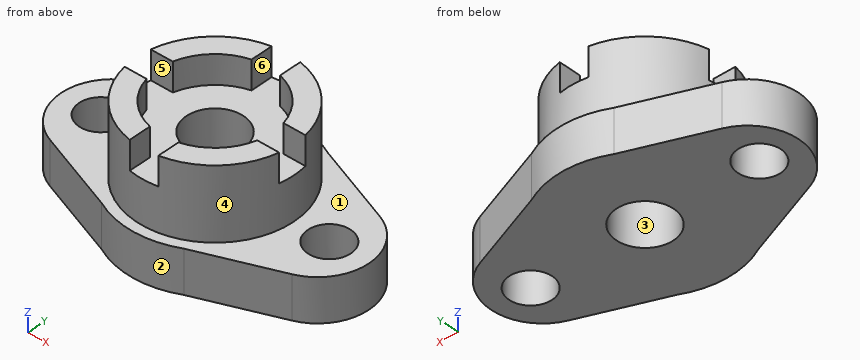
```python
from build123d import *

# Parameters (mm, degrees)
F1_DEPTH = 19.05
F2_DEPTH = 38.1
F3_R     = 34.925
F3_R_2   = 12.7
F4_DEPTH = 12.7
F6_DEPTH = 12.7
F0_R     = 9.525
F7_DEPTH = 19.05
F8_DEPTH = 103.378
F9_DEPTH = 38.1


# Not quite as in the source:
# - a feature names something its author has since deleted; it is built from what else it names


with BuildPart() as f1:
    # F0 (on Top) → F1 (new body)
    with BuildSketch(Plane.XY):
        with BuildLine():
            ThreePointArc((-34.925, 0), (0, -34.925), (34.925, 0))
            Line((34.925, 0), (25.4, 0))
            ThreePointArc((25.4, 0), (0, -25.4), (-25.4, 0))
            Line((-25.4, 0), (-34.925, 0))
        make_face()
        with BuildLine():
            Line((25.4, 0), (34.925, 0))
            ThreePointArc((34.925, 0), (0, 34.925), (-34.925, 0))
            Line((-34.925, 0), (-25.4, 0))
            ThreePointArc((-25.4, 0), (0, 25.4), (25.4, 0))
        make_face()
    extrude(amount=F1_DEPTH)

    # F0 (on Top) → F2 (join)
    with BuildSketch(Plane.XY):
        with BuildLine():
            ThreePointArc((-34.925, 0), (0, -34.925), (34.925, 0))
            Line((34.925, 0), (25.4, 0))
            ThreePointArc((25.4, 0), (0, -25.4), (-25.4, 0))
            Line((-25.4, 0), (-34.925, 0))
        make_face()
        with BuildLine():
            Line((25.4, 0), (34.925, 0))
            ThreePointArc((34.925, 0), (0, 34.925), (-34.925, 0))
            Line((-34.925, 0), (-25.4, 0))
            ThreePointArc((-25.4, 0), (0, 25.4), (25.4, 0))
        make_face()
        with BuildLine():
            ThreePointArc((-25.4, 0), (0, -25.4), (25.4, 0))
            Line((25.4, 0), (12.7, 0))
            ThreePointArc((12.7, 0), (0, -12.7), (-12.7, 0))
            Line((-12.7, 0), (-25.4, 0))
        make_face()
        with BuildLine():
            Line((12.7, 0), (25.4, 0))
            ThreePointArc((25.4, 0), (0, 25.4), (-25.4, 0))
            Line((-25.4, 0), (-12.7, 0))
            ThreePointArc((-12.7, 0), (0, 12.7), (12.7, 0))
        make_face()
    extrude(amount=F2_DEPTH)

    # F3 (on face) → F4 (join)
    with BuildSketch(Plane.XY.offset(38.1)):
        Circle(F3_R)
        Circle(F3_R_2, mode=Mode.SUBTRACT)
    extrude(amount=F4_DEPTH)

    # F5 (on face) → F6 (cut)
    with BuildSketch(Plane.XY.offset(50.8)):
        with BuildLine():
            ThreePointArc((-24.5934442484, -6.35), (-25.4, 0), (-24.5934442484, 6.35))
            Line((-24.5934442484, 6.35), (-34.3428758988, 6.35))
            ThreePointArc((-34.3428758988, 6.35), (-34.925, 0), (-34.3428758988, -6.35))
            Line((-34.3428758988, -6.35), (-24.5934442484, -6.35))
        make_face()
        with BuildLine():
            Line((6.35, -34.3428758988), (6.35, -24.5934442484))
            ThreePointArc((6.35, -24.5934442484), (0, -25.4), (-6.35, -24.5934442484))
            Line((-6.35, -24.5934442484), (-6.35, -34.3428758988))
            ThreePointArc((-6.35, -34.3428758988), (0, -34.925), (6.35, -34.3428758988))
        make_face()
        with BuildLine():
            Line((34.3428758988, 6.35), (24.5934442484, 6.35))
            ThreePointArc((24.5934442484, 6.35), (25.1975542852, 3.2005090291), (25.4, 0))
            ThreePointArc((25.4, 0), (25.1975542852, -3.2005090291), (24.5934442484, -6.35))
            Line((24.5934442484, -6.35), (34.3428758988, -6.35))
            ThreePointArc((34.3428758988, -6.35), (34.7791644937, -3.1883133656), (34.925, 0))
            ThreePointArc((34.925, 0), (34.7791644937, 3.1883133656), (34.3428758988, 6.35))
        make_face()
        with BuildLine():
            ThreePointArc((-6.35, 24.5934442484), (0, 25.4), (6.35, 24.5934442484))
            Line((6.35, 24.5934442484), (6.35, 34.3428758988))
            ThreePointArc((6.35, 34.3428758988), (0, 34.925), (-6.35, 34.3428758988))
            Line((-6.35, 34.3428758988), (-6.35, 24.5934442484))
        make_face()
    extrude(amount=-F6_DEPTH, mode=Mode.SUBTRACT)

    # F0 (on Top) → F7 (join)
    with BuildSketch(Plane.XY):
        with BuildLine():
            Line((53.7687589873, 21.2442149995), (18.2328532376, 34.9850083733))
            ThreePointArc((18.2328532376, 34.9850083733), (0, 39.4510804423), (-18.2328532376, 34.9850083733))
            Line((-18.2328532376, 34.9850083733), (-53.7687589873, 21.2442149995))
            ThreePointArc((-53.7687589873, 21.2442149995), (-68.3312757395, 0), (-53.7687589873, -21.2442149995))
            Line((-53.7687589873, -21.2442149995), (-18.2328532376, -34.9850083733))
            ThreePointArc((-18.2328532376, -34.9850083733), (0, -39.4510804423), (18.2328532376, -34.9850083733))
            Line((18.2328532376, -34.9850083733), (53.7687589873, -21.2442149995))
            ThreePointArc((53.7687589873, -21.2442149995), (68.3312757395, 0), (53.7687589873, 21.2442149995))
        make_face()
        with Locations((-50.8, 0)):
            Circle(F0_R, mode=Mode.SUBTRACT)
        with BuildLine():
            ThreePointArc((-34.925, 0), (0, 34.925), (34.925, 0))
            ThreePointArc((34.925, 0), (0, -34.925), (-34.925, 0))
        make_face(mode=Mode.SUBTRACT)
        with BuildLine():
            ThreePointArc((60.325, 0), (50.8, -9.525), (41.275, 0))
            ThreePointArc((41.275, 0), (50.8, 9.525), (60.325, 0))
        make_face(mode=Mode.SUBTRACT)
    extrude(amount=F7_DEPTH)

    # F5 (on face) → F8 (cut)
    with BuildSketch(Plane.XY.offset(50.8)):
        with BuildLine():
            Line((6.35, 6.35), (6.35, 0))
            Line((6.35, 0), (6.35, -6.35))
            Line((6.35, -6.35), (24.5934442484, -6.35))
            ThreePointArc((24.5934442484, -6.35), (25.1975542852, -3.2005090291), (25.4, 0))
            ThreePointArc((25.4, 0), (25.1975542852, 3.2005090291), (24.5934442484, 6.35))
            Line((24.5934442484, 6.35), (6.35, 6.35))
        make_face()
        with BuildLine():
            Line((-6.35, -6.35), (-6.35, 0))
            Line((-6.35, 0), (-6.35, 6.35))
            Line((-6.35, 6.35), (-24.5934442484, 6.35))
            ThreePointArc((-24.5934442484, 6.35), (-25.4, 0), (-24.5934442484, -6.35))
            Line((-24.5934442484, -6.35), (-6.35, -6.35))
        make_face()
        with BuildLine():
            Line((-6.35, 6.35), (0, 6.35))
            Line((0, 6.35), (6.35, 6.35))
            Line((6.35, 6.35), (6.35, 24.5934442484))
            ThreePointArc((6.35, 24.5934442484), (0, 25.4), (-6.35, 24.5934442484))
            Line((-6.35, 24.5934442484), (-6.35, 6.35))
        make_face()
        with BuildLine():
            Line((6.35, -6.35), (0, -6.35))
            Line((0, -6.35), (-6.35, -6.35))
            Line((-6.35, -6.35), (-6.35, -24.5934442484))
            ThreePointArc((-6.35, -24.5934442484), (0, -25.4), (6.35, -24.5934442484))
            Line((6.35, -24.5934442484), (6.35, -6.35))
        make_face()
        with BuildLine():
            Line((6.35, 24.5934442484), (6.35, 6.35))
            Line((6.35, 6.35), (24.5934442484, 6.35))
            ThreePointArc((24.5934442484, 6.35), (17.9605122421, 17.9605122421), (6.35, 24.5934442484))
        make_face()
        with BuildLine():
            Line((24.5934442484, -6.35), (6.35, -6.35))
            Line((6.35, -6.35), (6.35, -24.5934442484))
            ThreePointArc((6.35, -24.5934442484), (17.9605122421, -17.9605122421), (24.5934442484, -6.35))
        make_face()
        with BuildLine():
            Line((-24.5934442484, 6.35), (-6.35, 6.35))
            Line((-6.35, 6.35), (-6.35, 24.5934442484))
            ThreePointArc((-6.35, 24.5934442484), (-17.9605122421, 17.9605122421), (-24.5934442484, 6.35))
        make_face()
        with BuildLine():
            Line((-6.35, -24.5934442484), (-6.35, -6.35))
            Line((-6.35, -6.35), (-24.5934442484, -6.35))
            ThreePointArc((-24.5934442484, -6.35), (-17.9605122421, -17.9605122421), (-6.35, -24.5934442484))
        make_face()
    extrude(amount=-F8_DEPTH, mode=Mode.SUBTRACT)

    # F0 (on Top) → F9 (join)
    with BuildSketch(Plane.XY):
        with BuildLine():
            ThreePointArc((-25.4, 0), (0, -25.4), (25.4, 0))
            Line((25.4, 0), (12.7, 0))
            ThreePointArc((12.7, 0), (0, -12.7), (-12.7, 0))
            Line((-12.7, 0), (-25.4, 0))
        make_face()
        with BuildLine():
            Line((12.7, 0), (25.4, 0))
            ThreePointArc((25.4, 0), (0, 25.4), (-25.4, 0))
            Line((-25.4, 0), (-12.7, 0))
            ThreePointArc((-12.7, 0), (0, 12.7), (12.7, 0))
        make_face()
    extrude(amount=F9_DEPTH)


solid = f1.part
```
Design review of the part built by this model. Coordinates are the model's own, in mm. Face numbers are marked on the shaded views. A direction names the side the tool comes from. Coordinates: 2 decimals unless noted, no trailing zeros. Write each loop counter-clockwise with the first axis right and the second up, starting at its lowest first coordinate (ties: lowest second). Pieces come first, ordered by that corner, then holes. Notation, with made-up numbers: M 63.5,79.5 L 68.5,79.5 A25 ccw 68.5,114.5 Z; hole C -13,31 d10. An arc over 180 degrees is marked long. Answer as a JSON object with one key per item and string values.
Item 1: Add section B-B, the plane x = 0. Give the boundary of the cut face in (y, z) (3 decimals).
Outcome:
{"outline": "M -39.451,0 L -12.7,0 L -12.7,38.1 L -34.925,38.1 L -34.925,19.05 L -39.451,19.05 Z; M 12.7,0 L 39.451,0 L 39.451,19.05 L 34.925,19.05 L 34.925,38.1 L 12.7,38.1 Z"}
Item 2: Draft analysis for pull direction X (two halves, no side actions). For the marked faces 1, 2 and 3, state which applies: pulls with the +X half, pulls with the -X half, needs draft (parallel to the pull), parting line crosses it, or undercut.
Outcome:
{"face 1": "needs draft", "face 2": "parting line crosses it", "face 3": "undercut"}
Item 3: Insertion check: pin 1 Ø1.5 at (x, z) = (1, 37.5) entering from -Y; pin 2 Ø10.5 at (x, z) = (27.5, 43.5) entering from +Y; pin 3 Ø5 at (x, z) = (18, 14) entering from +Y; pin 4 Ø1.5 at (x, y) = (-27.5, -23.5) entering from -Z. Each pin has a flat end and moves straight along its axis. Give the tip position at first contact, or say it passes through.
Outcome:
{"pin 1": "y = -34.92", "pin 2": "y = 26.92", "pin 3": "y = 36.28", "pin 4": "z = 0"}
Item 4: Wall thickness on probe 1 along Y at (x, z) = (0, 13); probe 2 along Y at (x, z) = (0, 27) (3 decimals); probe 3 along Z at (x, y) = (18, -1.5): over which ranges is each line inside the solid? List them lowest first.
Outcome:
{"probe 1": "-39.45 to -12.7, 12.7 to 39.45", "probe 2": "-34.925 to -12.7, 12.7 to 34.925", "probe 3": "0 to 38.1"}
Item 5: Add section A-A, the plane z = 11.5. Give the boundary of the cut face in (x, y) (3 decimals), and give its area (3 significant figures).
Outcome:
{"outline": "M -53.769,-21.244 L -18.233,-34.985 A39.451 ccw 18.233,-34.985 L 53.769,-21.244 A22.777 ccw 53.769,21.244 L 18.233,34.985 A39.451 ccw -18.233,34.985 L -53.769,21.244 A22.777 ccw Z; hole C -50.8,0 d19.05; hole C 0,0 d25.4; hole C 50.8,0 d19.05", "area": "6,590 mm²"}
Item 6: Machinability: for the marked faces 4, 5 and 6, which of the approach directions +Z, -Z, +X, -X, +Y, -Y give a long, thin tool a straight path to every point of the face, cutting with its end or side? Answer none if there is none.
Outcome:
{"face 4": "+Z", "face 5": "+Z, +X, -X", "face 6": "+Z, +Y, -Y"}
Item 7: Add section D-D, the plane z = 36. Give the boundary of the cut face in (x, y) (3 decimals).
Outcome:
{"outline": "C 0,0 d69.85; hole C 0,0 d25.4"}
Item 8: Add section C-C, the plane y = 0. Give the boundary of the cut face in (x, z) (3 decimals), and give its area (3 significant figures).
Outcome:
{"outline": "M -68.331,0 L -60.325,0 L -60.325,19.05 L -68.331,19.05 Z; M -41.275,0 L -12.7,0 L -12.7,38.1 L -34.925,38.1 L -34.925,19.05 L -41.275,19.05 Z; M 12.7,0 L 41.275,0 L 41.275,19.05 L 34.925,19.05 L 34.925,38.1 L 12.7,38.1 Z; M 60.325,0 L 68.331,0 L 68.331,19.05 L 60.325,19.05 Z", "area": "2,240 mm²"}
